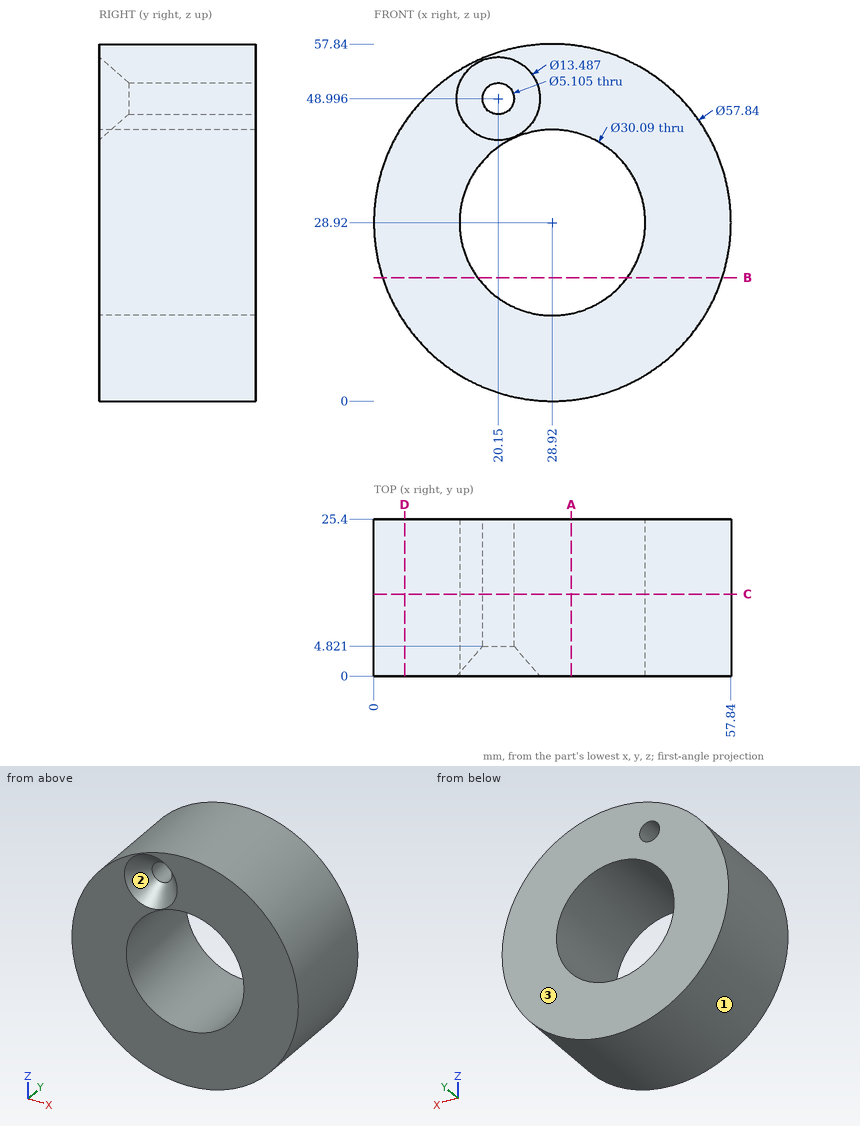
Study the drawing (mm; zero at the part's minimum x, y, z) and answer. Coordinates: 2 decimals unless noted, no trailing zeros. Loops run counter-clockwise (first coordinate to the right, second up) from the corner with the lowest first, then second, coordinate; pieces in that order, holes last. Notation, with made-up numbers: M 27,74 L 56,74 A32 cw 56,103 Z; hole C 52.5,-14 d4. An arc over 180 degrees is marked long. Answer as a JSON object with one key per item and string values. Group by question number.
Item 1: Section D-D (x = 5) is taken. Write down the section's boundary in (y, z) (1 decimal), and give its area (3 significant figures).
Item 2: Each of these flat-tipped pins is pushed along its axis until it touches: P1, Ø1.5, axis at y = 20.5, z = 29.5, coming from the -X side; P2, Ø8, axis at y = 8, z = 44, coming from the -X side; P3, Ø3, axis at x = 20.15, z = 49, coming from the +Y side; P4, Ø5, axis at x = 50, y = 3.5, coming from the +Z side. Where does it stop, or does it pass through?
Item 3: Determine the mould class of the marked faces 1, 2 and 3 for opening direction Z: +Z half, -Z half, draft (parallel to the pull), parting line (faces both ways), or undercut.
Item 4: Section C-C (y = 13.25) is taken. Give the number of separate pieces and of enclosed holes in the cut face, and give its area (3 significant figures).
Item 5: Section A-A (x = 32) is taken. Write down the section's boundary in (y, z) (1 decimal), and give its area (3 significant figures).
Item 6: Consider L1, parallel to Z at x = 28.5, y = 16.5; L2, parallel to Z at x = 23.5, y = 21 (1 decimal); L3, parallel to X at y = 14.5, z = 49 (1 decimal). Determine where each line is inside the solid, lowest interval first.
Item 7: Section B-B (z = 20) is taken. Write down the section's boundary in (x, y) (1 decimal).
Solved:
{
 "1": {"outline": "M 0,12.7 L 25.4,12.7 L 25.4,45.2 L 0,45.2 Z", "area": "826 mm2"},
 "2": {"P1": "stops at x = 0", "P2": "stops at x = 2.21", "P3": "passes through", "P4": "stops at z = 51.08"},
 "3": {"face 1": "parting line", "face 2": "undercut", "face 3": "draft"},
 "4": {"separate pieces": "1", "enclosed holes": "2", "area": "1,900 mm2"},
 "5": {"outline": "M 0,0.2 L 25.4,0.2 L 25.4,14.2 L 0,14.2 Z; M 0,43.6 L 25.4,43.6 L 25.4,57.7 L 0,57.7 Z", "area": "713 mm2"},
 "6": {"L1": "z = 0 to 13.88, 43.96 to 57.84", "L2": "z = 0.5 to 14.9, 43 to 57.3", "L3": "x = 8.1 to 17.6, 22.7 to 49.7"},
 "7": {"outline": "M 1.4,0 L 16.8,0 L 16.8,25.4 L 1.4,25.4 Z; M 41,0 L 56.4,0 L 56.4,25.4 L 41,25.4 Z"}
}
